Verification items for the finished model (mm, model axes). Face numbers are marked on the shaded views. A direction names the side the tool comes from. Give positions to 0.01 mm unless a question says otherwise; leave off trailing zeros. Write each loop counter-clockwise with the first axis right and the second up, starting at its lowest first coordinate (ties: lowest second). Pieces come first, ordered by that corner, then holes. Notation, with made-up numbers: (5.25, -12.5) -> (13.25, -12.5) arc R12 ccw to (13.25, -6.5) -> close; hole circle Ø1 at (20, 14). An arc over 180 degrees is marked (long way). Answer as CSV lines item,"result".
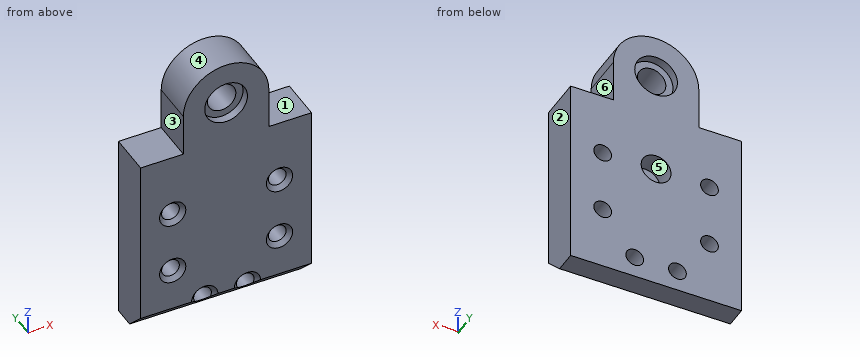
```python
from build123d import *

# Parameters (mm, degrees)
F0_W         = 40
F0_H         = 40
F0_R         = 2.074
F1_DEPTH     = 10
F2_W         = 10
F2_H         = 5
F3_DEPTH     = 10
F4_SIZE      = 1
F5_R         = 3.3235
F6_DEPTH     = 10.001
F7_R         = 5
F7_R_2       = 3.3235
F8_DEPTH     = 2
F10_R        = 3.5
F11_DEPTH    = 5
F12_T1_DEPTH = 65.7168298797


# Not quite as in the source:
# - a fillet or chamfer that OpenCascade refuses, or shapes differently, is made with other operations: its cross-section is extruded or revolved along the edge and cut away or added
# - a pattern or mirror of a feature is missing from the dataset's text; its kind, count and spacing are read off the source's solid


with BuildPart() as f1:
    # F0 (on Front) → F1 (new body)
    with BuildSketch(Plane.XZ):
        Rectangle(F0_W, F0_H)
        with Locations((-5, -15)):
            Circle(F0_R, mode=Mode.SUBTRACT)
        with Locations((-12.5, -5)):
            Circle(F0_R, mode=Mode.SUBTRACT)
        with Locations((5, -15)):
            Circle(F0_R, mode=Mode.SUBTRACT)
        with Locations((12.5, -5)):
            Circle(F0_R, mode=Mode.SUBTRACT)
        with Locations((-12.5, 10)):
            Circle(F0_R, mode=Mode.SUBTRACT)
        with Locations((12.5, 10)):
            Circle(F0_R, mode=Mode.SUBTRACT)
    extrude(amount=F1_DEPTH)

    # F2 (on face) → F3 (join, through all)
    with BuildSketch(Plane.XZ.offset(10)):
        with BuildLine():
            Line((10, 25), (10, 35))
            ThreePointArc((10, 35), (0, 45), (-10, 35))
            Line((-10, 35), (-10, 25))
            Line((-10, 25), (-10, 20))
            Line((-10, 20), (10, 20))
            Line((10, 20), (10, 25))
        make_face()
        with Locations((-15, 22.5)):
            Rectangle(F2_W, F2_H)
        with Locations((15, 22.5)):
            Rectangle(F2_W, F2_H)
    extrude(amount=-F3_DEPTH)

    # F4
    f4_edges = [f1.edges().sort_by_distance(p)[0] for p in [
        (-7.074, -10, -15),
        (2.926, -10, -15),
        (-14.574, -10, 10),
        (-14.574, -10, -5),
        (10.426, -10, -5),
        (10.426, -10, 10),
    ]]
    chamfer(f4_edges, length=F4_SIZE)

    # F5 (on face) → F6 (cut, through all)
    with BuildSketch(Plane.XZ.offset(10)):
        with Locations((0, 35)):
            Circle(F5_R)
    extrude(amount=-F6_DEPTH, mode=Mode.SUBTRACT)

    # F7 (on face) → F8 (cut)
    with BuildSketch(Plane.XZ.offset(10)):
        with Locations((0, 35)):
            Circle(F7_R)
        with Locations((0, 35)):
            Circle(F7_R_2, mode=Mode.SUBTRACT)
    f8 = extrude(amount=-F8_DEPTH, mode=Mode.SUBTRACT)

    # F8_copies: F8 across plane
    add(f8.mirror(Plane.ZX.offset(-5)), mode=Mode.SUBTRACT)

    # F10 (on face) → F11 (cut)
    with BuildSketch(Plane(origin=(0, 0, 0), x_dir=(-1, 0, 0), z_dir=(0, 1, 0))):
        with Locations((0, 10.311)):
            Circle(F10_R)
    extrude(amount=-F11_DEPTH, mode=Mode.SUBTRACT)

    # F12: chamfer of 5 on 1 edges, made by hand

    # F12_s2 → F12_t1 (cut)
    with BuildSketch(Plane.YZ.offset(-32.8584149398)):
        Polygon((-10, -15), (-5, -20), (-10, -20), align=None)
    extrude(amount=F12_T1_DEPTH, mode=Mode.SUBTRACT)


solid = f1.part
```
1) Draft check along Z on the marked faces 4, 5 and 6. Enter one of: +Z half, -Z half, draft (parallel to the pull), parting line (faces both ways), or undercut.
Reported:
face 4,"+Z half"
face 5,"undercut"
face 6,"draft"
2) Scan lines: line 1 along Z through (x, y) = (0, -3.7); line 2 along X through (y, z) = (-5, -15); line 3 along Z through (x, y) = (12.5, -3). Record each from-to range of solid material in increasing order.
Reported:
line 1,"-20 to 6.81, 13.81 to 31.68, 38.32 to 45"
line 2,"-20 to -7.07, -2.93 to 2.93, 7.07 to 20"
line 3,"-20 to -7.07, -2.93 to 7.93, 12.07 to 25"
3) Section check B-B (y = -7.25). Record the boundary of the cut face in (x, z).
Reported:
outline,"(-20, -17.75) -> (20, -17.75) -> (20, 25) -> (10, 25) -> (10, 35) arc R10 ccw to (-10, 35) -> (-10, 25) -> (-20, 25) -> close; hole circle Ø4.15 at (-12.5, -5); hole circle Ø4.15 at (-12.5, 10); hole circle Ø4.15 at (-5, -15); hole circle Ø6.65 at (0, 35); hole circle Ø4.15 at (5, -15); hole circle Ø4.15 at (12.5, -5); hole circle Ø4.15 at (12.5, 10)"
4) Section check C-C (x = 0). Record the boundary of the cut face in (y, z).
Reported:
outline,"(-10, -15) -> (-5, -20) -> (0, -20) -> (0, 6.81) -> (-5, 6.81) -> (-5, 13.81) -> (0, 13.81) -> (0, 30) -> (-2, 30) -> (-2, 31.68) -> (-8, 31.68) -> (-8, 30) -> (-10, 30) -> close; (-10, 40) -> (-8, 40) -> (-8, 38.32) -> (-2, 38.32) -> (-2, 40) -> (0, 40) -> (0, 45) -> (-10, 45) -> close"
5) Section check D-D (z = 37.5). Record the boundary of the cut face in (x, y), and give its area (3 significant figures).
Reported:
outline,"(-9.68, -10) -> (-4.33, -10) -> (-4.33, -8) -> (-2.19, -8) -> (-2.19, -2) -> (-4.33, -2) -> (-4.33, 0) -> (-9.68, 0) -> close; (2.19, -8) -> (4.33, -8) -> (4.33, -10) -> (9.68, -10) -> (9.68, 0) -> (4.33, 0) -> (4.33, -2) -> (2.19, -2) -> close"
area,"133 mm²"
6) Section check A-A (x = 12.5). Record the boundary of the cut face in (y, z).
Reported:
outline,"(-10, -15) -> (-5, -20) -> (0, -20) -> (0, -7.07) -> (-9, -7.07) -> (-10, -8.07) -> close; (-10, -1.93) -> (-9, -2.93) -> (0, -2.93) -> (0, 7.93) -> (-9, 7.93) -> (-10, 6.93) -> close; (-10, 13.07) -> (-9, 12.07) -> (0, 12.07) -> (0, 25) -> (-10, 25) -> close"
7) Tool access check on the marked faces 1, 2 and 3. Record the directions out of +Z, -Z, +X, -X, +Y, -Y that give a thin tool (end or side, any length) a straight path to the whole face; none if there is none.
Reported:
face 1,"+Z, +X, +Y, -Y"
face 2,"+Z, -Z, +X, +Y, -Y"
face 3,"+Z, -X, +Y, -Y"
8) Depth check by flat-ended pin: pin 1 (6.5 mm diameter, centred on x = 0, z = 10.311, fed in from +Y); pin 2 (5 mm diameter, centred on y = -3.5, z = 29, fed in from -X); pin 3 (9 mm diameter, centred on x = 0, z = 35, fed in from -Y). Enter the tip coordinate at first touch or a pass-through.
Reported:
pin 1,"y = -5"
pin 2,"x = -10"
pin 3,"y = -8"
